Check sheet for the modelled part. Datum: model origin and axes. Units: mm. A direction names the side the tool comes from. Round coordinates to 2 decimals unless told otherwise and drop trailing zeros. Loops run counter-clockwise (first coordinate to the right, second up) from the corner with the lowest first, then second, coordinate; pieces in that order, holes last. Notation, with made-up numbers: M 15,13.5 L 64,13.5 A28 cw 64,49.5 Z; hole C 48,14 d4. An arc over 180 degrees is marked long. Write item = value, one per line. Start each with the question number.
(1) Cross-section at D-D on z = -5.5. Record the boundary of the cut face in (x, y), plus the area to 3 significant figures.
(2) Go/stop test with flat-tipped pins: P1, Ø6.5, axis at x = 0, y = 0, coming from the -Z side; P2, Ø8, axis at x = -5.5, z = 2, coming from the +Y side; P3, Ø6, axis at y = 5.5, z = 2.5, coming from the -X side (3 decimals); P4, Ø4, axis at x = 0, y = -8.25, coming from the +Z side. Record where each tip stops, or that it passes through.
(3) Scan lines: L1, parallel to Y at x = 0, z = 0.9; L2, parallel to Y at x = 8.25, z = 2.15; L3, parallel to Z at x = 0.5, y = -6. Record each from-to range of solid material in increasing order. Write a range as from..to.
(4) Cross-section at C-C on x = -7.25. Record the boundary of the cut face in (y, z).
(5) Cross-section at A-A on x = 0. Record the boundary of the cut face in (y, z).
(6) Mould release check, pull along Y, two halves, no side actions. Record for faces 3 (the face through (-1.08, -4.88, -5.07)), 4 (the face through (-0.867, -3.905, -3.098)), 5 (the face through (5, -2, 0)), 6 (the face through (-9.75, 0.07, 1.52)): pulls with the +Y half, pulls with the -Y half, needs draft (parallel to the pull), parting line crosses it, or undercut.
(7) Cross-section at B-B on y = 8.25. Record the boundary of the cut face in (x, z).
(8) Set-up check for faces 1 (the face through (-1.08, -4.88, 3.49)), 2 (the face through (-1.5, 11.4, 1.5)): record each of +Z, -Z, +X, -X, +Y, -Y from which the full face is reachable in a straight line by a thin tool's end or side.
from build123d import *

# Parameters (mm, degrees)
SKETCH1_R                = 11.5
BOSS_EXTRUDE1_DEPTH      = 3
BOSS_EXTRUDE2_DEPTH      = 1
BOSS_EXTRUDE2_DEPTH_BACK = 13
SKETCH2_R                = 5
SKETCH2_R_2              = 4
SKETCH3_R                = 4
CUT_EXTRUDE1_DEPTH       = 5
SKETCH4_R                = 1.5
CUT_EXTRUDE2_DEPTH       = 5


with BuildPart() as part:
    # Sketch1 → Boss-Extrude1 (new body)
    with BuildSketch(Plane.XY):
        Circle(SKETCH1_R)
    extrude(amount=BOSS_EXTRUDE1_DEPTH)

    # Sketch2 → Boss-Extrude2 (add, two sides: drawn at the far end of the back side and taken through both)
    with BuildSketch(Plane.XY.offset(3).offset(-BOSS_EXTRUDE2_DEPTH_BACK)):
        Circle(SKETCH2_R)
        Circle(SKETCH2_R_2, mode=Mode.SUBTRACT)
    extrude(amount=BOSS_EXTRUDE2_DEPTH + BOSS_EXTRUDE2_DEPTH_BACK)

    # Sketch3 → Cut-Extrude1 (cut)
    with BuildSketch(Plane.XY.offset(3)):
        Circle(SKETCH3_R)
    extrude(amount=-CUT_EXTRUDE1_DEPTH, mode=Mode.SUBTRACT)

    # Sketch4 → Cut-Extrude2 (cut)
    with BuildSketch(Plane.XY.offset(3)):
        with Locations((0, 8.25)):
            Circle(SKETCH4_R)
        with Locations((8.25, 0)):
            Circle(SKETCH4_R)
        with Locations((0, -8.25)):
            Circle(SKETCH4_R)
        with Locations((-8.25, 0)):
            Circle(SKETCH4_R)
    extrude(amount=-CUT_EXTRUDE2_DEPTH, mode=Mode.SUBTRACT)


solid = part.part
Result:
q1.outline = C 0,0 d10; hole C 0,0 d8
q1.area = 28.3 mm^2
q2.P1 = through
q2.P2 = 11.4
q2.P3 = -11.225
q2.P4 = 3
q3.L1 = -11.5..-9.75, -6.75..-4, 4..6.75, 9.75..11.5
q3.L2 = -8.01..-1.5, 1.5..8.01
q3.L3 = 0..3
q4.outline = M -8.93,0 L -1.12,0 L -1.12,3 L -8.93,3 Z; M 1.12,0 L 8.93,0 L 8.93,3 L 1.12,3 Z
q5.outline = M -11.5,0 L -9.75,0 L -9.75,3 L -11.5,3 Z; M -6.75,0 L -5,0 L -5,-10 L -4,-10 L -4,4 L -5,4 L -5,3 L -6.75,3 Z; M 4,-10 L 5,-10 L 5,0 L 6.75,0 L 6.75,3 L 5,3 L 5,4 L 4,4 Z; M 9.75,0 L 11.5,0 L 11.5,3 L 9.75,3 Z
q6.face_3 = parting line crosses it
q6.face_4 = undercut
q6.face_5 = needs draft
q6.face_6 = undercut
q7.outline = M -8.01,0 L -1.5,0 L -1.5,3 L -8.01,3 Z; M 1.5,0 L 8.01,0 L 8.01,3 L 1.5,3 Z
q8.face_1 = +Z
q8.face_2 = +Z, -Z
